Design review of the part built by this model. Coordinates are the model's own, in mm. A direction names the side the tool comes from. Coordinates: 2 decimals unless noted, no trailing zeros. Write each loop counter-clockwise with the first axis right and the second up, starting at its lowest first coordinate (ties: lowest second). Pieces come first, ordered by that corner, then holes. Notation, with made-up numbers: (38.5, 31.25) - (72.5, 31.25) arc R24 cw to (72.5, 44.25) - close; hole circle Ø6 at (51, 80.5). An arc over 180 degrees is marked (long way). Use a Markdown table: item, result.
Autodesk Fusion 360 part; units mm, degrees
sketch "Sketch1" plane through (0, 0, 0) normal (0, 1, 0) x (1, 0, 0)
  line L0 (0, 0) -> (0, -32)
  line L1 (0, -32) -> (15, -32)
  line L2 (15, -32) -> (15, -22)
  line L3 (15, -22) -> (5, -22)
  line L4 (5, -22) -> (5, -5)
  line L5 (5, -5) -> (15, -5)
  line L6 (15, -5) -> (15, 0)
  line L7 (15, 0) -> (0, 0)
  dimension "d1" = 15
  dimension "d2" = 32
  dimension "d3" = 10
  dimension "d4" = 17
  dimension "d5" = 10
  dimension "d7" = 15
extrude "Extrude1" add sketch "Sketch1" along normal blind 40
fillet "Fillet1" radius 5 1 edges at (15, 20, 0)
fillet "Fillet2" radius 4 1 edges at (0, 20, 0)
fillet "Fillet3" radius 5 1 edges at (0, 20, 32)
equation "d2 = 17 mm + 10 mm + 5 mm"
(1) For pin 1 (5 mm diameter, centred on y = 20.5, z = 12, fed in from +X), flat-tipped, find the tip position at first contact; note if it passes through.
Determined:
| item | result |
|---|---|
| pin 1 | x = 5 |
(2) Machinability: for faces 1 (the flat face through (10, 20, 22)), 2 (the flat face through (0, 20, 15)), which of the approach directions +Z, -Z, +X, -X, +Y, -Y give a long, thin tool a straight path to every point of the face, cutting with its end or side? Answer none if there is none.
Determined:
| item | result |
|---|---|
| face 1 | +X, +Y, -Y |
| face 2 | +Z, -Z, -X, +Y, -Y |
(3) Take a section at A-A on x = 6.25. Write out the cut boundary in (y, z).
Determined:
| item | result |
|---|---|
| outline | (0, 0) - (40, 0) - (40, 5) - (0, 5) - close; (0, 22) - (40, 22) - (40, 32) - (0, 32) - close |
(4) Take a section at D-D on z = 12. Write out the cut boundary in (x, y), and give its area (3 significant figures).
Determined:
| item | result |
|---|---|
| outline | (0, 0) - (5, 0) - (5, 40) - (0, 40) - close |
| area | 200 mm2 |
(5) For L1, parallel to Z at x = 7.75, y = 14; L2, parallel to X at y = 31.5, z = 6; L3, parallel to Z at x = 12.75, y = 37.5, list the stretches that pass through material, from the lowest coordinate up. Write a range as from..to.
Determined:
| item | result |
|---|---|
| L1 | 0..5, 22..32 |
| L2 | 0..5 |
| L3 | 0.82..5, 22..32 |
(6) Take a section at C-C on x = 12. Write out the cut boundary in (y, z).
Determined:
| item | result |
|---|---|
| outline | (0, 0.42) - (40, 0.42) - (40, 5) - (0, 5) - close; (0, 22) - (40, 22) - (40, 32) - (0, 32) - close |
